For this review, take the finished solid that the model builds, in its own axes (mm). A direction names the side the tool comes from. Round coordinates to 2 decimals unless told otherwise and drop trailing zeros. Write each loop counter-clockwise with the first axis right and the second up, starting at its lowest first coordinate (ties: lowest second). Pieces come first, ordered by that corner, then holes.
from build123d import *

# Parameters (mm, degrees)
SKETCH1_ONE_SIDE_W   = 1.5
SKETCH1_ONE_SIDE_H   = 3
SKETCH1_ONE_SIDE_H_2 = 5
SKETCH1_ONE_SIDE_W_2 = 1
SKETCH1_ONE_SIDE_W_3 = 20
CHAMFER1_SIZE        = 1


with BuildPart() as part:
    # Sketch1 one side → Revolve4 (revolve)
    with BuildSketch(Plane(origin=(0, 0, 0), x_dir=(0, 0, -1), z_dir=(1, 0, 0))):
        with BuildLine():
            Line((-8, 0), (8, 0))
            ThreePointArc((8, 0), (2.070552361, 7.72740661), (-6.92820323, 4))
            ThreePointArc((-6.92820323, 4), (-7.72740661, 2.070552361), (-8, 0))
        make_face()
        with BuildLine():
            ThreePointArc((-8, 0), (-7.72740661, 2.070552361), (-6.92820323, 4))
            Line((-6.92820323, 4), (-13.5, 5))
            Line((-13.5, 5), (-13.5, 0))
            Line((-13.5, 0), (-8, 0))
        make_face()
        with Locations((-14.25, 6.5)):
            Rectangle(SKETCH1_ONE_SIDE_W, SKETCH1_ONE_SIDE_H)
        with Locations((-14.25, 2.5)):
            Rectangle(SKETCH1_ONE_SIDE_W, SKETCH1_ONE_SIDE_H_2)
        with Locations((-15.5, 2.5)):
            Rectangle(SKETCH1_ONE_SIDE_W_2, SKETCH1_ONE_SIDE_H_2)
        with Locations((-26, 2.5)):
            Rectangle(SKETCH1_ONE_SIDE_W_3, SKETCH1_ONE_SIDE_H_2)
    revolve(axis=Axis((0, 0, -8), (0, 0, -1)))

    # Chamfer1
    chamfer1_edges = [part.edges().sort_by_distance(p)[0] for p in [
        (0, -5, 36),
    ]]
    chamfer(chamfer1_edges, length=CHAMFER1_SIZE)


solid = part.part
(1) We need section D-D, the plane z = 31. Give the boundary of the cut face in (x, y).
Geometry check:
outline: circle Ø10 at (0, 0)
(2) Mouldability with a two-part tool opening along Z and no side actions: class faces 4 (the face through (0, 0, 36)), 5 (the face through (-4.88, -1.08, 25.14)), 6 (the face through (0.19, -4.39, 9.53)) as pulls with the +Z half, pulls with the -Z half, needs draft (parallel to the pull), parting line crosses it, or undercut.
Geometry check:
face 4: pulls with the +Z half
face 5: needs draft
face 6: undercut
(3) For line 1 along Z through (x, y) = (6.25, 0); line 2 along X through (y, z) = (0, 26.5); line 3 along Z through (x, y) = (-6.5, -3.5), list the stretches that pass through material, from the lowest coordinate up.
Geometry check:
line 1: z = -4.99 to 4.99, 13.5 to 15
line 2: x = -5 to 5
line 3: z = -3.08 to 3.08, 13.5 to 15
(4) We need section B-B, the plane y = 6.75. Give the boundary of the cut face in (x, z), and give its area (3 significant figures).
Geometry check:
outline: circle Ø8.59 at (0, 0); (-4.29, 13.5) - (4.29, 13.5) - (4.29, 15) - (-4.29, 15) - close
area: 70.8 mm2
(5) We need section A-A, the plane y = 0. Give the boundary of the cut face in (x, z).
Geometry check:
outline: (-8, 13.5) - (-5, 13.5) - (-4, 6.93) arc R8 ccw (long way) to (4, 6.93) - (5, 13.5) - (8, 13.5) - (8, 15) - (5, 15) - (5, 35) - (4, 36) - (-4, 36) - (-5, 35) - (-5, 15) - (-8, 15) - close
(6) For pin 1 Ø5 at (x, z) = (-4, 19.5) entering from +Y; pin 2 Ø8 at (x, y) = (6, 5.5) entering from +Z; pin 3 Ø3 at (y, z) = (-2.5, 30.5) entering from +X, all flat-tipped, find the tip position at first contact; note any pin that passes through.
Geometry check:
pin 1: stops at y = 4.77
pin 2: stops at z = 35.86
pin 3: stops at x = 4.9
(7) For faces 1 (the face through (-7.81, -1.73, 14.24)), 2 (the face through (-5.2, -0.1, 15)), 3 (the face through (-5.2, 0.1, 13.5)), list the 3-axis set-ups (+Z, -Z, +X, -X, +Y, -Y) from which the entire face can be reached by the end or side of a thin tool; tool diameter is ignored.
Geometry check:
face 1: +Z, -Z
face 2: +Z
face 3: none
